Can you work these out from the model? Positions are in its coordinate system, mm. A direction names the side the tool comes from. Give positions to 0.01 mm unless a question says otherwise; leave off trailing zeros. Order: outer loops, then holes, each group sorted by start corner. A loop starts at its lowest first (then second) coordinate and runs counter-clockwise, first axis right, second up. Notation, with made-up numbers: (-1, -30) - (36, -30) arc R22 cw to (36, -17) - close; hole circle Ø5 at (24.5, -9.5). An arc over 180 degrees is marked (long way). Answer as CSV lines item,"result".
```python
from build123d import *

# Parameters (mm, degrees)
F0_R      = 52.5
F0_R_2    = 48.8
F1_DEPTH  = 29
F2_R      = 52.5
F2_R_2    = 4
F3_DEPTH  = 5
F4_R      = 6.35
F4_R_2    = 4
F5_DEPTH  = 30
F7_R      = 6.85
F7_R_2    = 5.35
F8_DEPTH  = 1
F9_R      = 9.525
F9_R_2    = 4.384096
F10_DEPTH = 1
F11_R     = 5
F13_DEPTH = 25


with BuildPart() as f1:
    # F0 (on Front) → F1 (new body)
    with BuildSketch(Plane.XZ):
        Circle(F0_R)
        Circle(F0_R_2, mode=Mode.SUBTRACT)
    extrude(amount=F1_DEPTH)

    # F2 (on face) → F3 (join)
    with BuildSketch(Plane.XZ.offset(29)):
        Circle(F2_R)
        Circle(F2_R_2, mode=Mode.SUBTRACT)
    extrude(amount=F3_DEPTH)

    # F4 (on face) → F5 (join)
    with BuildSketch(Plane(origin=(0, -29, 0), x_dir=(-1, 0, 0), z_dir=(0, 1, 0))):
        Circle(F4_R)
        Circle(F4_R_2, mode=Mode.SUBTRACT)
    extrude(amount=F5_DEPTH)

    # F7 (on offset) → F8 (cut)
    with BuildSketch(Plane(origin=(0, -5, 0), x_dir=(-1, 0, 0), z_dir=(0, 1, 0))):
        Circle(F7_R)
        Circle(F7_R_2, mode=Mode.SUBTRACT)
    extrude(amount=-F8_DEPTH, mode=Mode.SUBTRACT)

    # F9 (on face) → F10 (join)
    with BuildSketch(Plane(origin=(0, -29, 0), x_dir=(-1, 0, 0), z_dir=(0, 1, 0))):
        Circle(F9_R)
        Circle(F9_R_2, mode=Mode.SUBTRACT)
    extrude(amount=F10_DEPTH)

    # F11
    f11_edges = [f1.edges().sort_by_distance(p)[0] for p in [
        (-52.5, -34, 0),
    ]]
    fillet(f11_edges, radius=F11_R)

    # F12 (on face) → F13 (cut)
    with BuildSketch(Plane.XZ.offset(34)):
        with BuildLine():
            ThreePointArc((42.598049, -8.812276), (43.5, 0), (42.598049, 8.812276))
            ThreePointArc((42.598049, 8.812276), (40.705485, 11.451793), (37.478164, 11.81682))
            Line((37.478164, 11.81682), (15.124019, 4.768585))
            ThreePointArc((15.124019, 4.768585), (11.627548, 0), (15.124019, -4.768585))
            Line((15.124019, -4.768585), (37.478164, -11.81682))
            ThreePointArc((37.478164, -11.81682), (40.705485, -11.451793), (42.598049, -8.812276))
        make_face()
        with BuildLine():
            ThreePointArc((28.93068, 32.484855), (21.75, 37.672105), (13.66737, 41.297131))
            ThreePointArc((13.66737, 41.297131), (10.435199, 40.977881), (8.505416, 38.365452))
            Line((8.505416, 38.365452), (3.432294, 15.482077))
            ThreePointArc((3.432294, 15.482077), (5.813774, 10.069752), (11.691725, 10.713492))
            Line((11.691725, 10.713492), (28.972748, 26.548632))
            ThreePointArc((28.972748, 26.548632), (30.270287, 29.526088), (28.93068, 32.484855))
        make_face()
        with BuildLine():
            ThreePointArc((-13.66737, 41.297131), (-21.75, 37.672105), (-28.93068, 32.484855))
            ThreePointArc((-28.93068, 32.484855), (-30.270287, 29.526088), (-28.972748, 26.548632))
            Line((-28.972748, 26.548632), (-11.691725, 10.713492))
            ThreePointArc((-11.691725, 10.713492), (-5.813774, 10.069752), (-3.432294, 15.482077))
            Line((-3.432294, 15.482077), (-8.505416, 38.365452))
            ThreePointArc((-8.505416, 38.365452), (-10.435199, 40.977881), (-13.66737, 41.297131))
        make_face()
        with BuildLine():
            ThreePointArc((-42.598049, 8.812276), (-43.5, 0), (-42.598049, -8.812276))
            ThreePointArc((-42.598049, -8.812276), (-40.705485, -11.451793), (-37.478164, -11.81682))
            Line((-37.478164, -11.81682), (-15.124019, -4.768585))
            ThreePointArc((-15.124019, -4.768585), (-11.627548, 0), (-15.124019, 4.768585))
            Line((-15.124019, 4.768585), (-37.478164, 11.81682))
            ThreePointArc((-37.478164, 11.81682), (-40.705485, 11.451793), (-42.598049, 8.812276))
        make_face()
        with BuildLine():
            ThreePointArc((-28.93068, -32.484855), (-21.75, -37.672105), (-13.66737, -41.297131))
            ThreePointArc((-13.66737, -41.297131), (-10.435199, -40.977881), (-8.505416, -38.365452))
            Line((-8.505416, -38.365452), (-3.432294, -15.482077))
            ThreePointArc((-3.432294, -15.482077), (-5.813774, -10.069752), (-11.691725, -10.713492))
            Line((-11.691725, -10.713492), (-28.972748, -26.548632))
            ThreePointArc((-28.972748, -26.548632), (-30.270287, -29.526088), (-28.93068, -32.484855))
        make_face()
        with BuildLine():
            ThreePointArc((13.66737, -41.297131), (21.75, -37.672105), (28.93068, -32.484855))
            ThreePointArc((28.93068, -32.484855), (30.270287, -29.526088), (28.972748, -26.548632))
            Line((28.972748, -26.548632), (11.691725, -10.713492))
            ThreePointArc((11.691725, -10.713492), (5.813774, -10.069752), (3.432294, -15.482077))
            Line((3.432294, -15.482077), (8.505416, -38.365452))
            ThreePointArc((8.505416, -38.365452), (10.435199, -40.977881), (13.66737, -41.297131))
        make_face()
    extrude(amount=-F13_DEPTH, mode=Mode.SUBTRACT)


solid = f1.part
```
1) If we mould it in two halves opening along Z, with no side actions, what happens to faces 1 (the cylindrical face through (50.076, -14.297, 15.77)), 2 (the cylindrical face through (-40.66, -31.54, 11.48)), 3 (the flat face through (-1.3, 1, -4.1))? For each: +Z half, -Z half, draft (parallel to the pull), parting line (faces both ways), or undercut.
Answer block:
face 1,"parting line"
face 2,"undercut"
face 3,"draft"
2) I need wall thicknesses on line 1 along Z through (x, y) = (0, -20.25); line 2 along Z through (x, y) = (-1, -24.5); line 3 along X through (y, z) = (-32, 33.5). Which ranges of each line are inside material? Lowest first, please. Write a range as [from, to].
Answer block:
line 1,"[-52.5, -48.8], [-6.35, -4], [4, 6.35], [48.8, 52.5]"
line 2,"[-52.49, -48.79], [-6.27, -3.87], [3.87, 6.27], [48.79, 52.49]"
line 3,"[-39.12, -27.75], [-7.43, 7.43], [27.75, 39.12]"
3) I'm going to push flat-ended pins straight in: P1, Ø3, axis at x = -4, y = -17.5, coming from the +Z side; P2, Ø1.5, axis at x = -27, z = 23, coming from the +Y side; P3, Ø12, axis at y = -20.5, z = -13, coming from the -X side. Where does each tip first touch, or does it pass through?
Answer block:
P1,"z = 52.44"
P2,"y = -29"
P3,"x = -52.03"
4) Which directions (+Z, -Z, +X, -X, +Y, -Y) give clear straight access to the entire face, cutting with the end or side of a thin tool? Please do faces 4 (the cylindrical face through (1.38, -17.15, -6.2)), 5 (the cylindrical face through (1.16, -5.493, -5.223)), 6 (the cylindrical face through (-21.86, -31.54, -37.61)).
Answer block:
face 4,"+Y"
face 5,"none"
face 6,"+Y, -Y"
5) I want a section at C-C on z = 0. Count the separate pieces of the cut face and the enclosed holes in it, plus the area to 3 significant figures.
Answer block:
separate pieces,"4"
enclosed holes,"0"
area,"515 mm2"
6) I want a section at B-B on y = -8. Write out the boundary of the cut face in (x, z).
Answer block:
outline,"circle Ø105 at (0, 0); circle Ø12.7 at (0, 0); hole circle Ø97.6 at (0, 0); hole circle Ø8 at (0, 0)"
